from build123d import *

# Parameters (mm, degrees)
SKETCH1_W           = 328.676
SKETCH1_H           = 100.076
SKETCH1_W_2         = 327.152
SKETCH1_H_2         = 98.552
SKETCH1_W_3         = 323.977
SKETCH1_H_3         = 95.377
SKETCH1_W_4         = 318.897
SKETCH1_H_4         = 90.297
BOSS_EXTRUDE1_DEPTH = 2.54
SKETCH1_3_W         = 328.676
SKETCH1_3_H         = 100.076
SKETCH1_3_W_2       = 327.152
SKETCH1_3_H_2       = 98.552
BOSS_EXTRUDE2_DEPTH = 12.065
SKETCH1_4_W         = 327.152
SKETCH1_4_H         = 98.552
SKETCH1_4_W_2       = 323.977
SKETCH1_4_H_2       = 95.377
BOSS_EXTRUDE3_DEPTH = 10.3505
SKETCH1_5_W         = 323.977
SKETCH1_5_H         = 95.377
SKETCH1_5_W_2       = 318.897
SKETCH1_5_H_2       = 90.297
BOSS_EXTRUDE4_DEPTH = 5.2832
SKETCH2_R           = 1.99999981
SKETCH2_R_2         = 1.130554
BOSS_EXTRUDE5_DEPTH = 2.9972
FILLET1_R           = 4.7625
FILLET2_R           = 1.5875
CUT_EXTRUDE1_DEPTH  = 1.5875
SKETCH4_R           = 4.7625
CUT_EXTRUDE2_DEPTH  = 173.050880012
CUT_EXTRUDE3_DEPTH  = 12.7
CUT_EXTRUDE4_START  = -1.58
CUT_EXTRUDE4_DEPTH  = 6.6473
SKETCH7_R           = 4.826
CUT_EXTRUDE5_DEPTH  = 1.27


with BuildPart() as part:
    # Sketch1 → Boss-Extrude1 (new body)
    # profile 1 of 4: a face of its own
    with BuildSketch(Plane.XY):
        Rectangle(SKETCH1_W, SKETCH1_H)
        Rectangle(SKETCH1_W_2, SKETCH1_H_2, mode=Mode.SUBTRACT)
    # profile 2 of 4: a face of its own
    with BuildSketch(Plane.XY):
        Rectangle(SKETCH1_W_2, SKETCH1_H_2)
        Rectangle(SKETCH1_W_3, SKETCH1_H_3, mode=Mode.SUBTRACT)
    # profile 3 of 4: a face of its own
    with BuildSketch(Plane.XY):
        Rectangle(SKETCH1_W_3, SKETCH1_H_3)
    # profile 4 of 4: a face of its own
    with BuildSketch(Plane.XY):
        Rectangle(SKETCH1_W_4, SKETCH1_H_4)
    extrude(amount=BOSS_EXTRUDE1_DEPTH)

    # Sketch1<3> → Boss-Extrude2 (add)
    with BuildSketch(Plane.XY):
        Rectangle(SKETCH1_3_W, SKETCH1_3_H)
        Rectangle(SKETCH1_3_W_2, SKETCH1_3_H_2, mode=Mode.SUBTRACT)
    extrude(amount=BOSS_EXTRUDE2_DEPTH)

    # Sketch1<4> → Boss-Extrude3 (add)
    with BuildSketch(Plane.XY):
        Rectangle(SKETCH1_4_W, SKETCH1_4_H)
        Rectangle(SKETCH1_4_W_2, SKETCH1_4_H_2, mode=Mode.SUBTRACT)
    extrude(amount=BOSS_EXTRUDE3_DEPTH)

    # Sketch1<5> → Boss-Extrude4 (add)
    with BuildSketch(Plane.XY):
        Rectangle(SKETCH1_5_W, SKETCH1_5_H)
        Rectangle(SKETCH1_5_W_2, SKETCH1_5_H_2, mode=Mode.SUBTRACT)
    extrude(amount=BOSS_EXTRUDE4_DEPTH)

    # Sketch2 → Boss-Extrude5 (add)
    # profile 1 of 6: a face of its own
    with BuildSketch(Plane.XY.offset(2.54)):
        with Locations((142.875, -28.575)):
            Circle(SKETCH2_R)
        with Locations((142.875, -28.575)):
            Circle(SKETCH2_R_2, mode=Mode.SUBTRACT)
    # profile 2 of 6: a face of its own
    with BuildSketch(Plane.XY.offset(2.54)):
        with Locations((142.875, 28.575)):
            Circle(SKETCH2_R)
        with Locations((142.875, 28.575)):
            Circle(SKETCH2_R_2, mode=Mode.SUBTRACT)
    # profile 3 of 6: a face of its own
    with BuildSketch(Plane.XY.offset(2.54)):
        with Locations((-42.8625, 0)):
            Circle(SKETCH2_R)
        with Locations((-42.8625, 0)):
            Circle(SKETCH2_R_2, mode=Mode.SUBTRACT)
    # profile 4 of 6: a face of its own
    with BuildSketch(Plane.XY.offset(2.54)):
        with Locations((33.3375, 0)):
            Circle(SKETCH2_R)
        with Locations((33.3375, 0)):
            Circle(SKETCH2_R_2, mode=Mode.SUBTRACT)
    # profile 5 of 6: a face of its own
    with BuildSketch(Plane.XY.offset(2.54)):
        with Locations((-142.875, 28.575)):
            Circle(SKETCH2_R)
        with Locations((-142.875, 28.575)):
            Circle(SKETCH2_R_2, mode=Mode.SUBTRACT)
    # profile 6 of 6: a face of its own
    with BuildSketch(Plane.XY.offset(2.54)):
        with Locations((-138.1125, -28.575)):
            Circle(SKETCH2_R)
        with Locations((-138.1125, -28.575)):
            Circle(SKETCH2_R_2, mode=Mode.SUBTRACT)
    extrude(amount=BOSS_EXTRUDE5_DEPTH)

    # Fillet1
    fillet1_edges = [part.edges().sort_by_distance(p)[0] for p in [
        (159.4485, 45.1485, 3.9116),
        (159.4485, -45.1485, 3.9116),
        (-159.4485, -45.1485, 3.9116),
        (-159.4485, 45.1485, 3.9116),
        (163.576, -49.276, 11.20775),
        (-163.576, -49.276, 11.20775),
        (-163.576, 49.276, 11.20775),
        (163.576, 49.276, 11.20775),
        (161.9885, 47.6885, 7.81685),
        (-161.9885, 47.6885, 7.81685),
        (-161.9885, -47.6885, 7.81685),
        (161.9885, -47.6885, 7.81685),
    ]]
    fillet(fillet1_edges, radius=FILLET1_R)

    # Fillet2
    fillet2_edges = [part.edges().sort_by_distance(p)[0] for p in [
        (-164.338, -50.038, 6.0325),
        (-164.338, 50.038, 6.0325),
        (164.338, 50.038, 6.0325),
        (164.338, -50.038, 6.0325),
    ]]
    fillet(fillet2_edges, radius=FILLET2_R)

    # Sketch3 → Cut-Extrude1 (cut)
    with BuildSketch(Plane(origin=(0, 0, 0), x_dir=(-1, 0, 0), z_dir=(0, 0, -1))):
        with BuildLine():
            Line((-26.9875, -15.875), (26.9875, -15.875))
            ThreePointArc((26.9875, -15.875), (29.23256403, -14.94506403), (30.1625, -12.7))
            Line((30.1625, -12.7), (30.1625, 12.7))
            ThreePointArc((30.1625, 12.7), (29.23256403, 14.94506403), (26.9875, 15.875))
            Line((26.9875, 15.875), (-26.9875, 15.875))
            ThreePointArc((-26.9875, 15.875), (-29.23256403, 14.94506403), (-30.1625, 12.7))
            Line((-30.1625, 12.7), (-30.1625, -12.7))
            ThreePointArc((-30.1625, -12.7), (-29.23256403, -14.94506403), (-26.9875, -15.875))
        make_face()
    extrude(amount=-CUT_EXTRUDE1_DEPTH, mode=Mode.SUBTRACT)

    # Sketch4 → Cut-Extrude2 (cut, through all)
    with BuildSketch(Plane.XY.offset(2.54)):
        Circle(SKETCH4_R)
    extrude(amount=-CUT_EXTRUDE2_DEPTH, mode=Mode.SUBTRACT)

    # Sketch5 → Cut-Extrude3 (cut)
    with BuildSketch(Plane(origin=(0, 50.038, 0), x_dir=(1, 0, 0), z_dir=(0, 1, 0))):
        with BuildLine():
            Line((145.765, -5.5372), (139.985, -5.5372))
            ThreePointArc((139.985, -5.5372), (138.151, -3.7032), (139.985, -1.8692))
            Line((139.985, -1.8692), (145.765, -1.8692))
            ThreePointArc((145.765, -1.8692), (147.599, -3.7032), (145.765, -5.5372))
        make_face()
    extrude(amount=-CUT_EXTRUDE3_DEPTH, mode=Mode.SUBTRACT)

    # Sketch6 → Cut-Extrude4 (cut)
    with BuildSketch(Plane.XY.offset(5.2832).offset(CUT_EXTRUDE4_START)):
        with BuildLine():
            Line((138.151, 45.1485), (147.599, 45.1485))
            Line((147.599, 45.1485), (147.599, 46.89475))
            ThreePointArc((147.599, 46.89475), (147.134032015, 48.017282015), (146.0115, 48.48225))
            Line((146.0115, 48.48225), (139.7385, 48.48225))
            ThreePointArc((139.7385, 48.48225), (138.615967985, 48.017282015), (138.151, 46.89475))
            Line((138.151, 46.89475), (138.151, 45.1485))
        make_face()
    extrude(amount=CUT_EXTRUDE4_DEPTH, mode=Mode.SUBTRACT)

    # Sketch7 → Cut-Extrude5 (cut)
    with BuildSketch(Plane(origin=(0, 0, 0), x_dir=(-1, 0, 0), z_dir=(0, 0, -1))):
        with Locations((-157.988, 43.688)):
            Circle(SKETCH7_R)
        with Locations((-157.988, -43.688)):
            Circle(SKETCH7_R)
        with Locations((157.988, -43.688)):
            Circle(SKETCH7_R)
        with Locations((157.988, 43.688)):
            Circle(SKETCH7_R)
    extrude(amount=-CUT_EXTRUDE5_DEPTH, mode=Mode.SUBTRACT)


solid = part.part
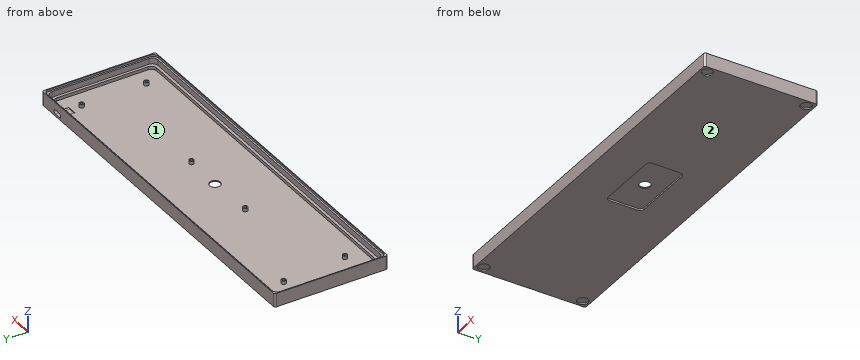
The listing builds one solid part. Answer for the finished solid, in the listing's coordinates (mm). Face numbers are marked on the shaded views. Round coordinates to 2 decimals unless told otherwise and drop trailing zeros. Loops run counter-clockwise (first coordinate to the right, second up) from the corner with the lowest first, then second, coordinate; pieces in that order, holes last. Notation, with made-up numbers: M 1,-8.75 L 33,-8.75 A24 cw 33,10.25 Z; hole C -10.75,84 d2. An arc over 180 degrees is marked long. Return JSON: item names as keys, results as strings.
Q1. Find section A-A, the plane x = 0. Determine the outline of the cut face in (y, z) (1 decimal).
Results list:
{"outline": "M -50,0 L -15.9,0 L -15.9,1.6 L -4.8,1.6 L -4.8,2.5 L -45.1,2.5 L -45.1,5.3 L -47.7,5.3 L -47.7,10.4 L -49.3,10.4 L -49.3,12.1 L -50,12.1 Z; M 4.8,1.6 L 15.9,1.6 L 15.9,0 L 50,0 L 50,12.1 L 49.3,12.1 L 49.3,10.4 L 47.7,10.4 L 47.7,5.3 L 45.1,5.3 L 45.1,2.5 L 4.8,2.5 Z"}
Q2. Each of these flat-tipped pins is pushed along its axis until it touches: pin 1 Ø8 at (x, y) = (115, -27) entering from +Z; pin 2 Ø2.5 at (x, y) = (-42.86, 0) entering from +Z; pin 3 Ø5 at (x, y) = (159.5, 43) entering from -Z. Where does it stop, or does it pass through?
Results list:
{"pin 1": "stops at z = 2.54", "pin 2": "stops at z = 5.54", "pin 3": "stops at z = 1.27"}
Q3. Find the intervals of material crossed by line 1 along Y through (x, z) = (-13.5, 10.5); line 2 along Y through (x, z) = (-29, 9.75); line 3 along X through (y, z) = (-30.5, 6.5), in increasing order. Write a range as from..to.
Results list:
{"line 1": "y = -50.04..-49.28, 49.28..50.04", "line 2": "y = -50.04..-47.69, 47.69..50.04", "line 3": "x = -164.34..-161.99, 161.99..164.34"}
Q4. Find section B-B, the plane x = 52. Determine the outline of the cut face in (y, z) (1 decimal), plus the area to 3 significant figures.
Results list:
{"outline": "M -50,0 L 50,0 L 50,12.1 L 49.3,12.1 L 49.3,10.4 L 47.7,10.4 L 47.7,5.3 L 45.1,5.3 L 45.1,2.5 L -45.1,2.5 L -45.1,5.3 L -47.7,5.3 L -47.7,10.4 L -49.3,10.4 L -49.3,12.1 L -50,12.1 Z", "area": "307 mm2"}
Q5. The mould has two halves that part along X. Classify the marked faces 1 and 2: released by +X, released by -X, zero draft, split by the parting line, or undercut.
Results list:
{"face 1": "undercut", "face 2": "zero draft"}
